```python
from build123d import *

# Parameters (mm, degrees)
F0_W     = 38.1
F0_H     = 25.4
F1_DEPTH = 50.8
F2_D     = 76.2


with BuildPart() as f1:
    # F0 (on Front) → F1 (new body)
    with BuildSketch(Plane.XZ):
        Polygon((-77.4996658967, 47.1252045367), (-77.4996658967, -23.9947954633), (-39.3996658967, -23.9947954633), (0.9780525733, -23.9947954633), (35.5579441879, -23.9947954633), (73.6579441879, -23.9947954633), (74.9003341033, -23.9947954633), (74.9003341033, 47.1252045367), (0, 47.1252045367), align=None)
        with Locations((-58.4496658967, -36.6947954633)):
            Rectangle(F0_W, F0_H)
        with BuildLine():
            ThreePointArc((0, 123.3252045367), (-54.7236774664, 101.4714986736), (-77.4996658967, 47.1252045367))
            Line((-77.4996658967, 47.1252045367), (0, 47.1252045367))
            Line((0, 47.1252045367), (0, 123.3252045367))
        make_face()
        with BuildLine():
            Line((0, 123.3252045367), (0, 47.1252045367))
            Line((0, 47.1252045367), (74.9003341033, 47.1252045367))
            ThreePointArc((74.9003341033, 47.1252045367), (53.0433148232, 100.5523958466), (0, 123.3252045367))
        make_face()
        with Locations((54.6079441879, -36.6947954633)):
            Rectangle(F0_W, F0_H)
    extrude(amount=F1_DEPTH)

    # F2 (through all)
    with Locations(Plane(origin=(0, 0, 0), x_dir=(1, 0, 0), z_dir=(0, 1, 0))):
        with Locations((-1.2996658967, -47.1362880764)):
            Hole(F2_D / 2)


solid = f1.part
```
Model file for the job. Use its own axes, mm. A direction names the side the tool comes from. Round coordinates to 2 decimals unless told otherwise and drop trailing zeros. Write each loop counter-clockwise with the first axis right and the second up, starting at its lowest first coordinate (ties: lowest second). Pieces come first, ordered by that corner, then holes. Notation, with made-up numbers: (-8, 2) - (-3, 2) arc R8 ccw to (-3, 15) - close; hole circle Ø4 at (80.5, 73). An arc over 180 degrees is marked (long way). One line per item, written item: value.
(1) Cut at D-D, the plane z = 97. Give the cut face in (x, y).
Values follow:
outline: (-58.92, -50.8) - (56.32, -50.8) - (56.32, 0) - (-58.92, 0) - close
(2) Drop flat-ended pins along their axis: P1, Ø1.4, axis at x = 74.5, y = -23, coming from the -Z side; P2, Ø3, axis at x = -37, y = -11, coming from the +Z side; P3, Ø7.5, axis at y = -24.5, z = -39, coming from the +X side. Give the stop position or say it passes through.
Values follow:
P1: stops at z = -23.99
P2: stops at z = 115.23
P3: stops at x = 73.66
(3) Cut at A-A, the plane z = -27.5. Give the cut face in (x, y), plus the area to 3 significant figures.
Values follow:
outline: (-77.5, -50.8) - (-39.4, -50.8) - (-39.4, 0) - (-77.5, 0) - close; (35.56, -50.8) - (73.66, -50.8) - (73.66, 0) - (35.56, 0) - close
area: 3,870 mm²
(4) Cut at C-C, the plane y = -44.5. Give the cut face in (x, z).
Values follow:
outline: (-77.5, -49.39) - (-39.4, -49.39) - (-39.4, -23.99) - (35.56, -23.99) - (35.56, -49.39) - (73.66, -49.39) - (73.66, -23.99) - (74.9, -23.99) - (74.9, 47.13) arc R76.2 ccw to (-77.5, 47.13) - close; hole circle Ø76.2 at (-1.3, 47.14)
(5) 3-axis set-ups, long thin cutter, end or side, ignore diameter. For faces 5 (the flat face through (-2, -50.8, 0)), 6 (the flat face through (-2, -25, -23.995)), 7 (the flat face through (73.658, -25, -37)): which of +Z, -Z, +X, -X, +Y, -Y reach the whole face in a straight line?
Values follow:
face 5: +Z, -Z, +X, -X, -Y
face 6: -Z, +Y, -Y
face 7: -Z, +X, +Y, -Y
(6) Cut at B-B, the plane x = 28. Give the cut face in (y, z).
Values follow:
outline: (-50.8, -23.99) - (0, -23.99) - (0, 22.78) - (-50.8, 22.78) - close; (-50.8, 71.49) - (0, 71.49) - (0, 117.48) - (-50.8, 117.48) - close
(7) Wall check: probe 1 along X at (y, z) = (-33.5, 48); probe 2 along Z at (x, y) = (-0.5, -2); probe 3 along Z at (x, y) = (1, -30.5). Give the ranges that are in metal, low to high.
Values follow:
probe 1: x = -77.49 to -39.39, 36.79 to 74.9
probe 2: z = -23.99 to 9.04, 85.23 to 123.33
probe 3: z = -23.99 to 9.11, 85.17 to 123.3
(8) Two-plate mould, pull along X, no slides. Class faces 1 (the flat face through (-39.4, -25, -37)), 2 (the flat face through (-59, -25, -49.395)), 3 (the flat face through (74.9, -25, 11)), 4 (the flat face through (35.558, -25, -37)): pulls with the +X half, pulls with the -X half, needs draft (parallel to the pull), parting line crosses it, or undercut.
Values follow:
face 1: undercut
face 2: needs draft
face 3: pulls with the +X half
face 4: undercut
